Geometry: final body of the model. Coordinates: model frame, mm. A direction names the side the tool comes from. Give positions to 0.01 mm unless a question says otherwise; leave off trailing zeros. Write each loop counter-clockwise with the first axis right and the second up, starting at its lowest first coordinate (ties: lowest second). Pieces come first, ordered by that corner, then holes.
Q1. Line query: L1, parallel to Y at x = -108.5, z = -6; L2, parallel to X at y = 6, z = 13; L3, parallel to Y at x = -60.5, z = -3. Output: solid intervals per line, ascending.
Q2. Reachability of faces 1 (the face through (9.466, 17.916, -10.538)), 2 (the face through (0, -10, 10)) from +Z, -Z, +X, -X, +Y, -Y: full face, straight path, thin tool, end or side. Return the list, or none.
Q3. Pin query (flat end, axial travel): pin 1 (8 mm diameter, centred on x = -96.5, y = -11, fed in from +Z); pin 2 (12 mm diameter, centred on x = -91.5, y = -12, fed in from +Z); pin 3 (10 mm diameter, centred on y = -11, z = -11, fed in from -X). Return the tip coordinate at first contact, or that it passes through.
Q4. Cut plane A-A on x = -43. Return the cut outline in (y, z).
```python
from build123d import *

# Parameters (mm, degrees)
BOSS_EXTRUDE2_DEPTH = 19.2
SKETCH3_R           = 12
BOSS_EXTRUDE3_DEPTH = 150
CHAMFER1_SIZE       = 2.4
SKETCH5_OUTSIDE_W   = 599.33
SKETCH5_OUTSIDE_H   = 605.76
SKETCH5_OUTSIDE_R   = 20.784609691
CUT_EXTRUDE1_DEPTH  = 150
CUT_EXTRUDE1_TAPER  = 60


with BuildPart() as part:
    # Sketch1 → Boss-Extrude2 (new body)
    with BuildSketch(Plane(origin=(0, 0, 0), x_dir=(0, 0, -1), z_dir=(1, 0, 0))):
        Polygon((0, 24), (-20.784609691, 12), (-20.784609691, -12), (0, -24), (20.784609691, -12), (20.784609691, 12), align=None)
    extrude(amount=BOSS_EXTRUDE2_DEPTH)

    # Sketch3 → Boss-Extrude3 (add)
    with BuildSketch(Plane.ZY):
        Circle(SKETCH3_R)
    extrude(amount=BOSS_EXTRUDE3_DEPTH)

    # Chamfer1
    chamfer1_edges = [part.edges().sort_by_distance(p)[0] for p in [
        (-150, 0, -12),
    ]]
    chamfer(chamfer1_edges, length=CHAMFER1_SIZE)

    # Sketch5 outside → Cut-Extrude1 (cut)
    with BuildSketch(Plane(origin=(19.2, 0, 0), x_dir=(0, 0, -1), z_dir=(1, 0, 0))):
        Rectangle(SKETCH5_OUTSIDE_W, SKETCH5_OUTSIDE_H)
        Circle(SKETCH5_OUTSIDE_R, mode=Mode.SUBTRACT)
    extrude(amount=-CUT_EXTRUDE1_DEPTH, taper=CUT_EXTRUDE1_TAPER, mode=Mode.SUBTRACT)


solid = part.part
```
Data:
1. L1: y = -10.39 to 10.39
1. L2: x = 0 to 19.2
1. L3: y = -11.62 to 11.62
2. face 1: -Z, +X, -X, +Y
2. face 2: -X
3. pin 1: stops at z = 9.75
3. pin 2: stops at z = 10.39
3. pin 3: stops at x = -149.04
4. outline: circle Ø24 at (0, 0)
